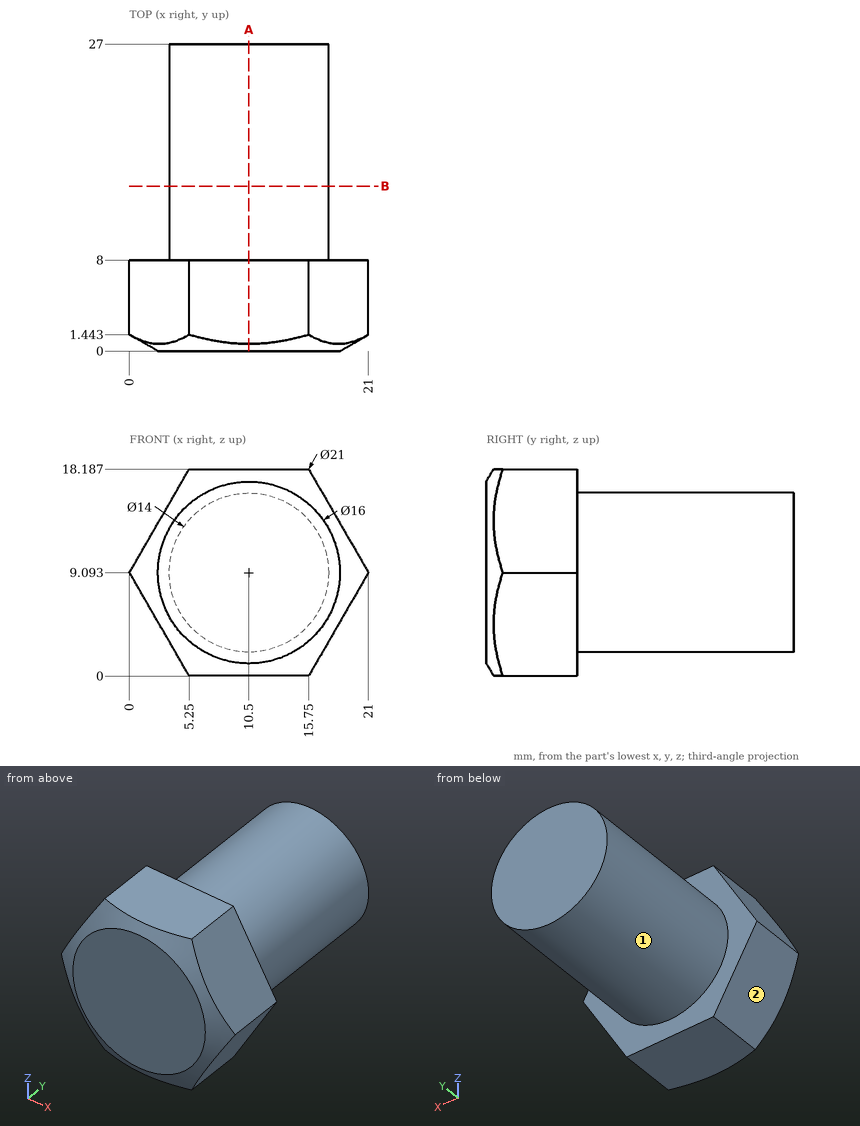
Source: three-view drawing plus pictorial views. Frame: mm from the lowest corner of the part. A direction names the side the tool comes from. Round coordinates to 2 decimals unless told otherwise and drop trailing zeros. Loops run counter-clockwise (first coordinate to the right, second up) from the corner with the lowest first, then second, coordinate; pieces in that order, holes last.
Item 1: Contact query for flat-ended pins moving along their axis: P1, Ø4, axis at x = 17.5, z = 16, coming from the +Y side; P2, Ø8, axis at x = 6, y = 14, coming from the -Z side; P3, Ø1, axis at x = 8, y = 17.5, coming from the +Z side. Output: stop coordinate, or through.
Checked values:
P1: stops at y = 8
P2: stops at z = 2.11
P3: stops at z = 15.8
Item 2: Line query: L1, parallel to Z at x = 10.75, y = 22.5; L2, parallel to Y at x = 5.25, z = 14; L3, parallel to Y at x = 15.75, z = 16.5. Output: solid intervals per line, ascending.
Checked values:
L1: z = 2.1 to 16.09
L2: y = 0 to 8
L3: y = 0.62 to 8
Item 3: Section B-B, the plane y = 14.5. Output: boundary loops of the cut face in (x, z), plus the area to 3 significant figures.
Checked values:
outline: circle Ø14 at (10.5, 9.09)
area: 154 mm2
Item 4: Reachability of the marked faces 1 and 2 from +Z, -Z, +X, -X, +Y, -Y: full face, straight path, thin tool, end or side. Return the list, or none.
Checked values:
face 1: +Y
face 2: -Z, -X, +Y, -Y
Item 5: Section A-A, the plane x = 10.5. Output: boundary loops of the cut face in (y, z), plus the area to 3 significant figures.
Checked values:
outline: (0, 1.09) - (0.63, 0) - (8, 0) - (8, 2.09) - (27, 2.09) - (27, 16.09) - (8, 16.09) - (8, 18.19) - (0.63, 18.19) - (0, 17.09) - close
area: 411 mm2
